Can you work these out from the model? Positions are in its coordinate system, mm. A direction names the side the tool comes from. Coordinates: 2 decimals unless noted, no trailing zeros. Loops run counter-clockwise (first coordinate to the right, second up) from the corner with the lowest first, then second, coordinate; pieces in that order, holes last. Notation, with made-up numbers: M 34,56.25 L 59,56.25 A17 cw 59,68.25 Z; hole C 82,-31 d7. An arc over 180 degrees is marked long. Answer as a JSON object with one key per item and string values. Group by question number.
Item 1: We'd pull the mould along X, two halves only. Please class faces 1 (the cylindrical face through (-11.662, -6.974, 0.986)), 2 (the flat face through (0.2, -5.5, 0)), 3 (the cylindrical face through (13.885, -7.949, 0.986)): +X half, -X half, draft (parallel to the pull), parting line (faces both ways), or undercut.
Item 2: Suppose I cut it at D-D (z = 1.5). Write out the boundary of the cut face in (x, y), then the cut area to 3 significant figures.
Item 3: If I drill on line 1 (Y direction, x = 1, z = 1.6); line 2 (X direction, y = 4.75, z = 0.9); line 3 (X direction, y = 3.5, z = 0.75), over which ranges is the centre line in solid material (lowest first)?
Item 4: Which directions (+Z, -Z, +X, -X, +Y, -Y) give clear straight access to the entire face, cutting with the end or side of a thin tool? Please do faces 4 (the flat face through (0, -5, 1)), 5 (the flat face through (0.2, -5.5, 2)).
Item 5: Suppose I cut it at C-C (y = -6). Write out the boundary of the cut face in (x, z), then the cut area to 3 significant figures.
Item 6: I'm going to push a flat-ended pin straight in: pin 1 Ø1 at (x, z) = (3.5, 0.5) entering from +Y. Where does the tip first touch, or does it pass through?
Item 7: Suppose I cut it at B-B (x = 0.25). Write out the boundary of the cut face in (y, z), then the cut area to 3 significant figures.
Item 8: Suppose I cut it at A-A (y = 2). Write out the boundary of the cut face in (x, z), then the cut area to 3 significant figures.
```python
from build123d import *

# Parameters (mm, degrees)
SKETCH_1_R      = 1.6
SKETCH_1_W      = 10
SKETCH_1_H      = 10
EXTRUDE_1_DEPTH = 2


with BuildPart() as part:
    # ｽｹｯﾁ1 → ﾎﾞｽ - 押し出し1 (new body)
    with BuildSketch(Plane.XY):
        with BuildLine():
            Line((-13.856406461, -4), (-3.464101615, 14))
            ThreePointArc((-3.464101615, 14), (0, 16), (3.464101615, 14))
            Line((3.464101615, 14), (13.856406461, -4))
            ThreePointArc((13.856406461, -4), (13.856406461, -8), (10.392304845, -10))
            Line((10.392304845, -10), (-10.392304845, -10))
            ThreePointArc((-10.392304845, -10), (-13.856406461, -8), (-13.856406461, -4))
        make_face()
        with Locations((0, 12)):
            Circle(SKETCH_1_R, mode=Mode.SUBTRACT)
        with Locations((10.392304845, -6)):
            Circle(SKETCH_1_R, mode=Mode.SUBTRACT)
        with Locations((-10.392304845, -6)):
            Circle(SKETCH_1_R, mode=Mode.SUBTRACT)
        Rectangle(SKETCH_1_W, SKETCH_1_H, mode=Mode.SUBTRACT)
    extrude(amount=EXTRUDE_1_DEPTH)


solid = part.part
```
From the geometry:
{
 "1": {"face 1": "undercut", "face 2": "draft", "face 3": "+X half"},
 "2": {"outline": "M -13.86,-4 A4 ccw -10.39,-10 L 10.39,-10 A4 ccw 13.86,-4 L 3.46,14 A4 ccw -3.46,14 Z; hole C -10.39,-6 d3.2; hole M -5,-5 L 5,-5 L 5,5 L -5,5 Z; hole C 0,12 d3.2; hole C 10.39,-6 d3.2", "area": "363 mm2"},
 "3": {"line 1": "-10 to -5, 5 to 10.75, 13.25 to 15.87", "line 2": "-8.8 to -5, 5 to 8.8", "line 3": "-9.53 to -5, 5 to 9.53"},
 "4": {"face 4": "+Z, -Z", "face 5": "+Z, +X, -X, +Y, -Y"},
 "5": {"outline": "M -14.39,0 L -11.99,0 L -11.99,2 L -14.39,2 Z; M -8.79,0 L 8.79,0 L 8.79,2 L -8.79,2 Z; M 11.99,0 L 14.39,0 L 14.39,2 L 11.99,2 Z", "area": "44.8 mm2"},
 "6": {"pin 1": "y = 14.65"},
 "7": {"outline": "M -10,0 L -5,0 L -5,2 L -10,2 Z; M 5,0 L 10.42,0 L 10.42,2 L 5,2 Z; M 13.58,0 L 15.99,0 L 15.99,2 L 13.58,2 Z", "area": "25.7 mm2"},
 "8": {"outline": "M -10.39,0 L -5,0 L -5,2 L -10.39,2 Z; M 5,0 L 10.39,0 L 10.39,2 L 5,2 Z", "area": "21.6 mm2"}
}
